Design review of the part built by this model. Coordinates are the model's own, in mm. Round coordinates to 2 decimals unless told otherwise and drop trailing zeros. Loops run counter-clockwise (first coordinate to the right, second up) from the corner with the lowest first, then second, coordinate; pieces in that order, holes last. Notation, with made-up numbers: (-9.75, -38.5) - (7.25, -38.5) arc R23 cw to (7.25, -8.5) - close; hole circle Ø2 at (-6, 22). An arc over 180 degrees is marked (long way). Answer as CSV lines item,"result". Start each with the question number.
(1) Consider section C-C (x = -35.5). Give the boundary of the cut face in (y, z).
(2) For P1, Ø15.5, axis at y = -7, z = 25.5, coming from the -X side; P2, Ø1.1, axis at x = -50.5, y = -9.5, coming from the +Z side; P3, Ø8, axis at y = 2.5, z = 34.5, coming from the -X side; P4, Ø8, axis at y = 9.5, z = 43.5, coming from the -X side, all flat-tipped, find the tip position at first contact; note any pin that passes through.
(3) Consider section B-B (y = 5.5). Give the boundary of the cut face in (x, z).
(4) Wall thickness on L1, parallel to Y at x = -25.5, z = 43.5; L2, parallel to Z at x = -18.5, y = -13.5; L3, parallel to X at y = 15.5, z = 43: over which ranges is each line inside the solid? List them lowest first.
(5) Consider section A-A (z = 44). Give the boundary of the cut face in (x, y).
(6) Consider section D-D (z = 12). Give the boundary of the cut face in (x, y), and give its area (3 significant figures).
from build123d import *

# Parameters (mm, degrees)
F0_W      = 34.5459179953
F0_H      = 84.0644203126
F1_DEPTH  = 2
F2_W      = 2
F2_H      = 84.0644203126
F3_DEPTH  = 50
F4_W      = 2
F4_H      = 84.0644203126
F5_DEPTH  = 50
F6_W      = 84.0644203126
F6_H      = 2.4206031561
F7_DEPTH  = 32.2
F8_W      = 30.5459179953
F8_H      = 2
F9_DEPTH  = 47.6
F10_R     = 5
F11_R     = 5
F12_W     = 2
F12_H     = 47.5793968439
F13_DEPTH = 31.3
F14_W     = 4.5
F14_H     = 32
F15_DEPTH = 25
F16_W     = 42.5153374672
F16_H     = 38
F17_DEPTH = 1
F18_R     = 3.3259647968
F19_DEPTH = 1
F20_R     = 0.99999
F22_DEPTH = 1


# Not quite as in the source:
# - a fillet or chamfer is up to 0.001 mm smaller than in the source, because OpenCascade refuses the exact size


with BuildPart() as f1:
    # F0 (on Top) → F1 (new body)
    with BuildSketch(Plane.XY):
        with Locations((-31.5246856771, -0.4831273109)):
            Rectangle(F0_W, F0_H)
    extrude(amount=F1_DEPTH)

    # F2 (on face) → F3 (join)
    with BuildSketch(Plane.XY.offset(2)):
        with Locations((-15.2517266795, -0.4831273109)):
            Rectangle(F2_W, F2_H)
    extrude(amount=F3_DEPTH)

    # F4 (on face) → F5 (join)
    with BuildSketch(Plane.XY.offset(2)):
        with Locations((-47.7976446748, -0.4831273109)):
            Rectangle(F4_W, F4_H)
    extrude(amount=F5_DEPTH)

    # F6 (on face) → F7 (join)
    with BuildSketch(Plane.YZ.offset(-46.7976446748)):
        with Locations((-0.4831273109, 50.789698422)):
            Rectangle(F6_W, F6_H)
    extrude(amount=F7_DEPTH)

    # F8 (on face) → F9 (join)
    with BuildSketch(Plane.XY.offset(2)):
        with Locations((-31.5246856771, 40.5490828454)):
            Rectangle(F8_W, F8_H)
    extrude(amount=F9_DEPTH)

    # F10
    f10_edges = [f1.edges().sort_by_distance(p)[0] for p in [
        (-31.524686, 41.549083, 52),
    ]]
    fillet(f10_edges, radius=F10_R)

    # F11
    f11_edges = [f1.edges().sort_by_distance(p)[0] for p in [
        (-31.524686, 41.549083, 0),
    ]]
    fillet(f11_edges, radius=F11_R)

    # F12 (on face) → F13 (join)
    with BuildSketch(Plane(origin=(-16.2517266795, 0, 0), x_dir=(0, -1, 0), z_dir=(-1, 0, 0))):
        with Locations((41.5153374672, 25.789698422)):
            Rectangle(F12_W, F12_H)
    extrude(amount=F13_DEPTH)

    # F14 (on face) → F15 (cut)
    with BuildSketch(Plane(origin=(-48.7976446748, 0, 0), x_dir=(0, -1, 0), z_dir=(-1, 0, 0))):
        with Locations((-19.0076687336, 26)):
            Rectangle(F14_W, F14_H)
    extrude(amount=-F15_DEPTH, mode=Mode.SUBTRACT)

    # F16 (on face) → F17 (join)
    with BuildSketch(Plane(origin=(-48.7976446748, 0, 0), x_dir=(0, -1, 0), z_dir=(-1, 0, 0))):
        with Locations((21.2576687336, 26)):
            Rectangle(F16_W, F16_H)
    extrude(amount=F17_DEPTH)

    # F18 (on face) → F19 (join)
    with BuildSketch(Plane(origin=(-49.7976446748, 0, 0), x_dir=(0, -1, 0), z_dir=(-1, 0, 0))):
        with Locations((10.0552504882, 26)):
            Circle(F18_R)
    extrude(amount=F19_DEPTH)

    # F20 (radius 1 in the source; OpenCascade refuses exactly that, so slightly less here)
    f20_edges = [f1.edges().sort_by_distance(p)[0] for p in [
        (-50.797645, -6.729286, 26),
    ]]
    fillet(f20_edges, radius=F20_R)

    # F21 (on face) → F22 (cut)
    with BuildSketch(Plane(origin=(-50.7976446748, 0, 0), x_dir=(0, -1, 0), z_dir=(-1, 0, 0))):
        Polygon((11.3802812994, 26.4259647968), (10.0552504882, 26.4259647968), (8.548588492, 26.4259647968), (8.548588492, 25.5740352032), (11.3802812994, 25.5740352032), align=None)
    extrude(amount=-F22_DEPTH, mode=Mode.SUBTRACT)


solid = f1.part
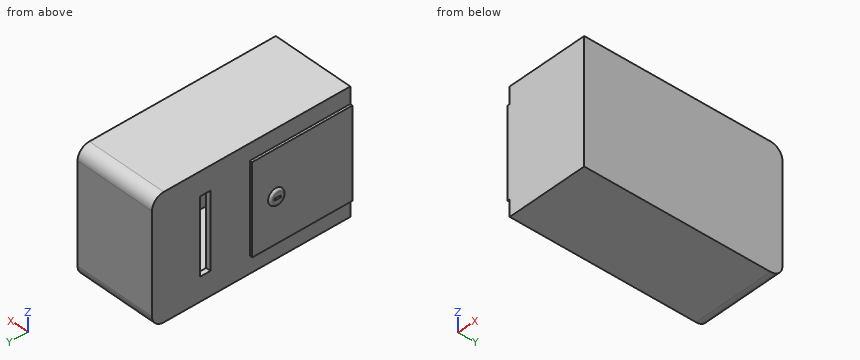
Determined:
1,outline,"(-42.52, 0) - (36.55, 0) arc R5 ccw to (41.55, 5) - (41.55, 47) arc R5 ccw to (36.55, 52) - (-42.52, 52) - close; hole (-40.52, 2) - (39.55, 2) - (39.55, 49.58) - (-40.52, 49.58) - close"
2,P1,"stops at x = -50.8"
2,P2,"stops at z = 29.29"
2,P3,"stops at x = -49.8"
2,P4,"stops at x = -48.8"
3,outline,"(-48.8, 0) - (-14.25, 0) - (-14.25, 52) - (-48.8, 52) - close; hole (-46.8, 2) - (-16.25, 2) - (-16.25, 49.58) - (-46.8, 49.58) - close"
4,L1,"y = -42.52 to -40.52, 39.55 to 41.55"
4,L2,"z = 0 to 2, 49.58 to 52"
4,L3,"x = -48.8 to -46.8, -16.25 to -14.25"
5,outline,"(-49.8, -42.52) - (-14.25, -42.52) - (-14.25, 41.55) - (-48.8, 41.55) - (-48.8, 0) - (-49.8, 0) - close; hole (-46.8, -40.52) - (-16.25, -40.52) - (-16.25, 39.55) - (-46.8, 39.55) - close"
6,outline,"(-49.8, -42.52) - (-14.25, -42.52) - (-14.25, 41.55) - (-48.8, 41.55) - (-48.8, 21.26) - (-46.8, 21.26) - (-46.8, 39.55) - (-16.25, 39.55) - (-16.25, -40.52) - (-46.8, -40.52) - (-46.8, 16.76) - (-48.8, 16.76) - (-48.8, 0) - (-49.8, 0) - close"
6,area,"492 mm^2"
